The drawing under review shows one solid part. Ordinate dimensions are in mm from its lowest x, y, z. A direction names the side the tool comes from. Coordinates: 2 decimals unless noted, no trailing zeros. Loops run counter-clockwise (first coordinate to the right, second up) from the corner with the lowest first, then second, coordinate; pieces in that order, holes last. Notation, with made-up numbers: (68.5, 7.25) -> (95.5, 7.25) arc R30 cw to (95.5, 33.25) -> close; hole circle Ø9 at (85, 45.5). An arc over 180 degrees is marked (long way). Use a Markdown table: item, result.
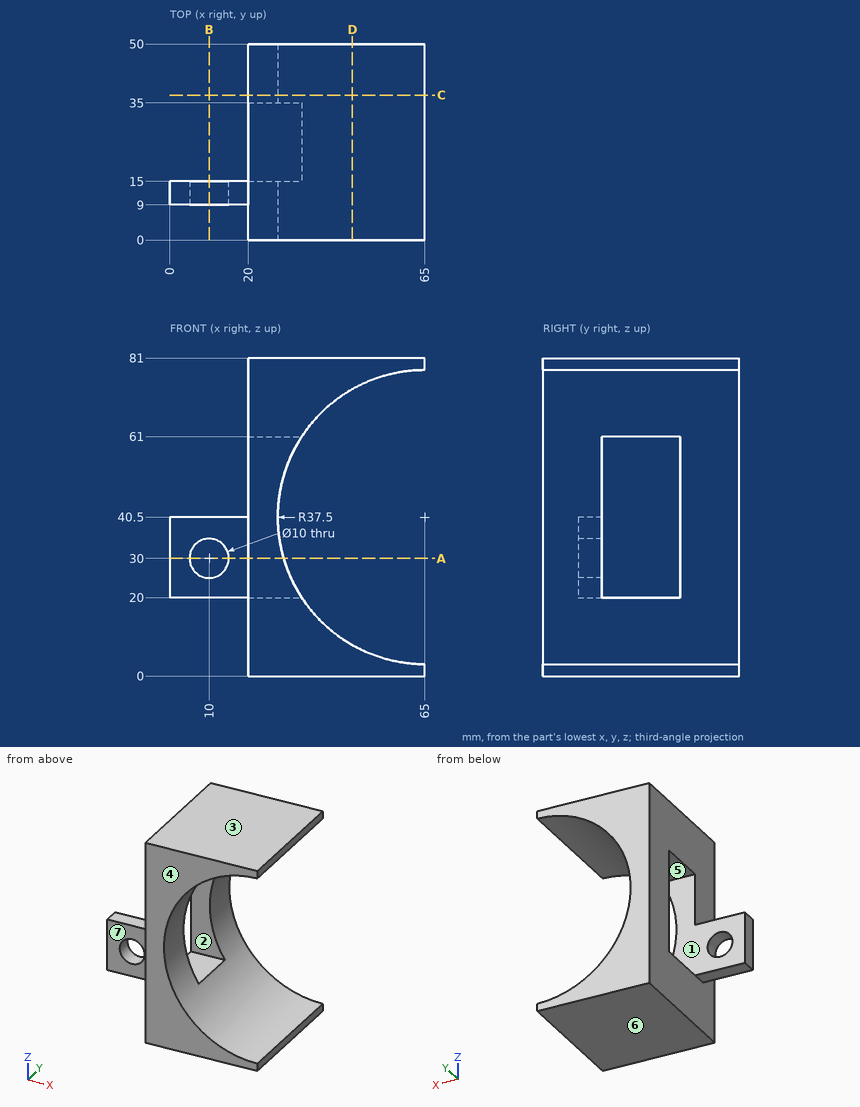
(1) Take a section at D-D on x = 46.5. Write out the cut boundary in (y, z).
Found:
| item | result |
|---|---|
| outline | (0, 0) -> (50, 0) -> (50, 7.88) -> (0, 7.88) -> close; (0, 73.12) -> (50, 73.12) -> (50, 81) -> (0, 81) -> close |
(2) Mouldability with a two-part tool opening along Z and no side actions: class the marked faces 1, 2, 3 and 4 as pulls with the +Z half, pulls with the -Z half, needs draft (parallel to the pull), parting line crosses it, or undercut.
Found:
| item | result |
|---|---|
| face 1 | undercut |
| face 2 | undercut |
| face 3 | pulls with the +Z half |
| face 4 | needs draft |
(3) Take a section at A-A on z = 30. Write out the cut boundary in (x, y).
Found:
| item | result |
|---|---|
| outline | (0, 9) -> (5, 9) -> (5, 15) -> (0, 15) -> close; (15, 9) -> (20, 9) -> (20, 0) -> (29, 0) -> (29, 15) -> (15, 15) -> close; (20, 35) -> (29, 35) -> (29, 50) -> (20, 50) -> close |
(4) For the marked faces 5, 6 and 7, list the 3-axis set-ups (+Z, -Z, +X, -X, +Y, -Y) from which the entire face can be reached by the end or side of a thin tool; tool diameter is ignored.
Found:
| item | result |
|---|---|
| face 5 | +X, -X |
| face 6 | -Z, +X, -X, +Y, -Y |
| face 7 | +Z, -Z, -X, -Y |
(5) For line 1 along Y through (x, z) = (21.5, 27); line 2 along Z through (x, y) = (32.5, 11); line 3 along Z through (x, y) = (35, 18.5), list the stretches that pass through material, from the lowest coordinate up.
Found:
| item | result |
|---|---|
| line 1 | y = 0 to 15, 35 to 50 |
| line 2 | z = 0 to 21.79, 59.21 to 81 |
| line 3 | z = 0 to 18, 63 to 81 |
(6) Take a section at B-B on x = 10. Write out the cut boundary in (y, z), plus the area to 3 significant figures.
Found:
| item | result |
|---|---|
| outline | (9, 20) -> (15, 20) -> (15, 25) -> (9, 25) -> close; (9, 35) -> (15, 35) -> (15, 40.5) -> (9, 40.5) -> close |
| area | 63.0 mm^2 |
(7) For pin 1 Ø11.5 at (x, z) = (10, 30) entering from +Y; pin 2 Ø6.5 at (x, y) = (9.5, 13.5) entering from +Z; pin 3 Ø1.8 at (x, y) = (6, 13) entering from -Z, all flat-tipped, find the tip position at first contact; note any pin that passes through.
Found:
| item | result |
|---|---|
| pin 1 | stops at y = 15 |
| pin 2 | stops at z = 40.5 |
| pin 3 | stops at z = 20 |
(8) Take a section at C-C on y = 37. Write out the cut boundary in (x, z).
Found:
| item | result |
|---|---|
| outline | (20, 0) -> (65, 0) -> (65, 3) arc R37.5 cw to (65, 78) -> (65, 81) -> (20, 81) -> close |
